Geometry check sheet. Reference: the model listing, model coordinates, mm. Face numbers are marked on the shaded views. A direction names the side the tool comes from. Round coordinates to 2 decimals unless told otherwise and drop trailing zeros. Loops run counter-clockwise (first coordinate to the right, second up) from the corner with the lowest first, then second, coordinate; pieces in that order, holes last.
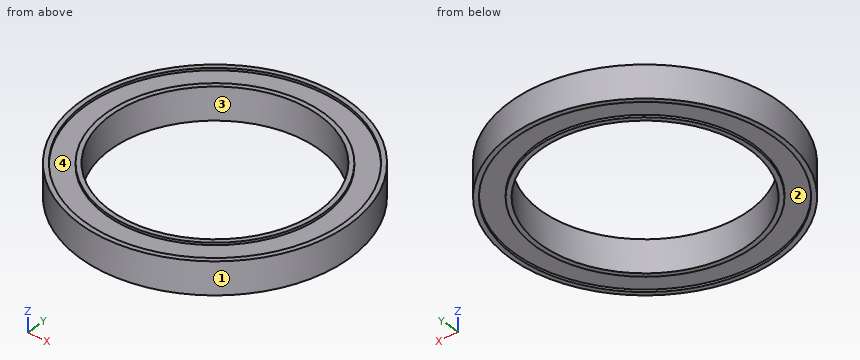
Autodesk Inventor part; units mm, degrees
ref_plane "YZ Plane" through (0, 0, 0) normal (1, 0, 0) x (0, 1, 0)
ref_plane "XZ Plane" through (0, 0, 0) normal (0, 1, 0) x (-1, 0, 0)
ref_plane "XY Plane" through (0, 0, 0) normal (0, 0, 1) x (1, 0, 0)
sketch "Sketch1" plane through (0, 0, 0) normal (0, 0, 1) x (1, 0, 0)
  circle A0 centre (0, 0) radius 29
  circle A1 centre (0, 0) radius 22.5
  dimension "d0" = 58
  dimension "d1" = 45
extrude "Extrusion1" add sketch "Sketch1" along normal blind 7
sketch "Sketch2" plane through (0, 0, 7) normal (0, 0, 1) x (1, 0, 0)
  circle A0 centre (0, 0) radius 29
  circle A1 centre (0, 0) radius 22.5
  circle A2 centre (0, 0) radius 28
  circle A3 centre (0, 0) radius 23.5
  dimension "d4" = 1
  dimension "d5" = 1
extrude "Extrusion2" cut sketch "Sketch2" against normal blind 0.5 contours A2
sketch "Sketch3" plane through (0, 0, 0) normal (0, 0, -1) x (-1, 0, 0)
  circle A0 centre (0, 0) radius 28
  circle A1 centre (0, 0) radius 23.5
extrude "Extrusion3" cut sketch "Sketch3" against normal blind 0.5
properties part number "bearing_58x45x7"
1) Gauge pin test, flat ends, axial feed: pin 1 (4 mm diameter, centred on x = -3.5, z = 3.5, fed in from +Y); pin 2 (4 mm diameter, centred on x = 9.5, y = -17.5, fed in from +Z); pin 3 (3 mm diameter, centred on y = 22.5, z = 4.5, fed in from -X); pin 4 (3 mm diameter, centred on y = -19.5, z = 4, fed in from +X). Record the tip position at first contact, or that the pin passes through.
Report:
pin 1: stops at y = 28.96
pin 2: passes through
pin 3: stops at x = -20
pin 4: stops at x = 22.74
2) Access from +Z, -Z, +X, -X, +Y, -Y to the whole of each face (thin tool, end or side, straight path). Record for the marked faces 3 and 4.
Report:
face 3: +Z, -Z
face 4: +Z
3) Mould release check, pull along X, two halves, no side actions. Record for the marked faces 1 and 2: +X half, -X half, draft (parallel to the pull), parting line (faces both ways), or undercut.
Report:
face 1: parting line
face 2: undercut
4) Sectioned sample at C-C, the plane z = 3.5. Record the cut outline in (x, y).
Report:
outline: circle Ø58 at (0, 0); hole circle Ø45 at (0, 0)
5) Scan lines: line 1 along Y through (x, z) = (0, 0.2); line 2 along Y through (x, z) = (-0.5, 3.25); line 3 along X through (y, z) = (-16, 0.75). Record each from-to range of solid material in increasing order.
Report:
line 1: y = -29 to -28, -23.5 to -22.5, 22.5 to 23.5, 28 to 29
line 2: y = -29 to -22.49, 22.49 to 29
line 3: x = -24.19 to -15.82, 15.82 to 24.19
6) Sectioned sample at A-A, the plane y = 0. Record the cut outline in (x, z), then the cut area to 3 significant figures.
Report:
outline: (-29, 0) - (-28, 0) - (-28, 0.5) - (-23.5, 0.5) - (-23.5, 0) - (-22.5, 0) - (-22.5, 7) - (-23.5, 7) - (-23.5, 6.5) - (-28, 6.5) - (-28, 7) - (-29, 7) - close; (22.5, 0) - (23.5, 0) - (23.5, 0.5) - (28, 0.5) - (28, 0) - (29, 0) - (29, 7) - (28, 7) - (28, 6.5) - (23.5, 6.5) - (23.5, 7) - (22.5, 7) - close
area: 82.0 mm2
